from build123d import *

# Parameters (mm, degrees)
SKETCH1_W             = 200
SKETCH1_H             = 215
EXTRUDE1_DEPTH        = 10
M8_TAPPED_HOLE1_D     = 6.8
M8_TAPPED_HOLE1_DEPTH = 19.75
M8_TAPPED_HOLE1_TIP   = 2.042926105
M8_TAPPED_HOLE2_D     = 6.8
M8_TAPPED_HOLE2_DEPTH = 19.75
M8_TAPPED_HOLE2_TIP   = 2.042926105
SKETCH5_R             = 50
EXTRUDE2_DEPTH        = 10
SKETCH6_R             = 50
EXTRUDE3_DEPTH        = 10
FILLET1_R             = 10
M6_TAPPED_HOLE1_D     = 5
M6_TAPPED_HOLE1_DEPTH = 8
M6_TAPPED_HOLE1_TIP   = 1.502151548


with BuildPart() as part:
    # Sketch1 → Extrude1 (new body)
    with BuildSketch(Plane(origin=(0, 0, 0), x_dir=(1, 0, 0), z_dir=(0, 1, 0))):
        Rectangle(SKETCH1_W, SKETCH1_H)
    extrude(amount=EXTRUDE1_DEPTH)

    # M8 Tapped Hole1
    with Locations(Plane(origin=(-60, 10, -16.5), x_dir=(0, 0, 1), z_dir=(0, 1, 0))):
        with Locations((0, 0), (0, 120), (68, 0), (68, 120)):
            Hole(M8_TAPPED_HOLE1_D / 2, depth=M8_TAPPED_HOLE1_DEPTH)
            with Locations((0, 0, -(M8_TAPPED_HOLE1_DEPTH + M8_TAPPED_HOLE1_TIP / 2))):  # 118° drill point
                Cone(0, M8_TAPPED_HOLE1_D / 2, M8_TAPPED_HOLE1_TIP, mode=Mode.SUBTRACT)

    # M8 Tapped Hole2
    with Locations(Plane(origin=(-15, 10, -97.5), x_dir=(0, 0, 1), z_dir=(0, 1, 0))):
        with Locations((0, 0), (40, 0), (40, 30), (0, 30)):
            Hole(M8_TAPPED_HOLE2_D / 2, depth=M8_TAPPED_HOLE2_DEPTH)
            with Locations((0, 0, -(M8_TAPPED_HOLE2_DEPTH + M8_TAPPED_HOLE2_TIP / 2))):  # 118° drill point
                Cone(0, M8_TAPPED_HOLE2_D / 2, M8_TAPPED_HOLE2_TIP, mode=Mode.SUBTRACT)

    # Sketch5 → Extrude2 (cut)
    with BuildSketch(Plane(origin=(0, 10, 0), x_dir=(1, 0, 0), z_dir=(0, 1, 0))):
        with Locations(Location((0, -17.5, 0), (0, 0, 270))):
            Circle(SKETCH5_R)
    extrude(amount=-EXTRUDE2_DEPTH, mode=Mode.SUBTRACT)

    # Sketch6 → Extrude3 (cut)
    with BuildSketch(Plane(origin=(0, 10, 0), x_dir=(1, 0, 0), z_dir=(0, 1, 0))):
        with Locations((0, 155.5)):
            Circle(SKETCH6_R)
    extrude(amount=-EXTRUDE3_DEPTH, mode=Mode.SUBTRACT)

    # Fillet1
    fillet1_edges = [part.edges().sort_by_distance(p)[0] for p in [
        (-100, 5, -107.5),
        (100, 5, -107.5),
        (100, 5, 107.5),
        (-100, 5, 107.5),
    ]]
    fillet(fillet1_edges, radius=FILLET1_R)

    # M6 Tapped Hole1
    with Locations(Plane(origin=(-56, 0, -38.5), x_dir=(0, 0, -1), z_dir=(0, -1, 0))):
        with Locations((0, 0), (0, 112), (-112, 0), (-112, 112)):
            Hole(M6_TAPPED_HOLE1_D / 2, depth=M6_TAPPED_HOLE1_DEPTH)
            with Locations((0, 0, -(M6_TAPPED_HOLE1_DEPTH + M6_TAPPED_HOLE1_TIP / 2))):  # 118° drill point
                Cone(0, M6_TAPPED_HOLE1_D / 2, M6_TAPPED_HOLE1_TIP, mode=Mode.SUBTRACT)


solid = part.part
Read the model definition and answer for the solid it produces. Units are mm, in the model's axes. A direction names the side the tool comes from. Round coordinates to 2 decimals unless told otherwise and drop trailing zeros. Order: outer loops, then holes, each group sorted by start corner. A loop starts at its lowest first (then second) coordinate and runs counter-clockwise, first axis right, second up. Notation, with made-up numbers: (32.25, -19) - (61.25, -19) arc R28 ccw to (61.25, 4) - close; hole circle Ø8 at (43, -7.75). An arc over 180 degrees is marked (long way). Use one line per item in the form item = value. Start each with the question number.
(1) Find the intervals of material crossed by line 1 along Z through (x, y) = (56, 5); line 2 along X through (y, z) = (4, 73.5); line 3 along Z through (x, y) = (-58.5, 9.5), in increasing order. Write a range as from..to.
(2) A flat-ended cylindrical pin translates along its axis: pin 1 Ø4 at (x, z) = (-56, -38.5) entering from -Y. Find the tip coordinate at first contact, or state that the pin passes through.
(3) For faces 4 (the face through (-1, 10, -49)), 5 (the face through (-56.96, 4.06, -36.19)), determine the directions among +Z, -Z, +X, -X, +Y, -Y from which every point of the face is accessible in a straight line to the end or side of a thin tool.
(4) The part is cut by section A-A (x = 0). Give the vertices of the cut face in (y, z).
(5) Determine the mould class of faces 1 (the face through (-97.15, 5.07, -104.49)), 2 (the face through (-1, 0, -49)), 3 (the face through (-17.069, 4.93, -94.802)) for opening direction X: +X half, -X half, draft (parallel to the pull), parting line (faces both ways), or undercut.
(6) The part is cut by section D-D (z = 18). Give the vertices of the cut face in (x, y).
(7) The part is cut by section C-C (y = 2.25). Count the separate pieces of the cut face and the enclosed holes in it, then the cut area to 3 significant figures.
(8) The part is cut by section B-B (z = -57.5). Give the vertices of the cut face in (x, y), then the cut area to 3 significant figures.
Checked values:
q1.line_1 = -107.5..-41, -36..71, 76..107.5
q1.line_2 = -100..-58.5, -53.5..53.5, 58.5..100
q1.line_3 = -107.5..-19.55, -13.45..48.45, 54.55..107.5
q2.pin_1 = 8.3
q3.face_4 = +Z, -Z, +X, -X, +Y
q3.face_5 = -Y
q4.outline = (0, -105.5) - (10, -105.5) - (10, -32.5) - (0, -32.5) - close; (0, 67.5) - (10, 67.5) - (10, 107.5) - (0, 107.5) - close
q5.face_1 = -X half
q5.face_2 = draft
q5.face_3 = undercut
q6.outline = (-100, 0) - (-50, 0) - (-50, 10) - (-100, 10) - close; (50, 0) - (100, 0) - (100, 10) - (50, 10) - close
q7.separate_pieces = 1
q7.enclosed_holes = 13
q7.area = 34,700 mm^2
q8.outline = (-100, 0) - (-18.4, 0) - (-18.4, 10) - (-100, 10) - close; (-11.6, 0) - (11.6, 0) - (11.6, 10) - (-11.6, 10) - close; (18.4, 0) - (100, 0) - (100, 10) - (18.4, 10) - close
q8.area = 1,860 mm^2
